Build history of the part. All positions in model axes, mm. Face numbers are marked on the shaded views. A direction names the side the tool comes from. Round coordinates to 2 decimals unless told otherwise and drop trailing zeros. Loops run counter-clockwise (first coordinate to the right, second up) from the corner with the lowest first, then second, coordinate; pieces in that order, holes last. Notation, with made-up numbers: M 7,5.5 L 55,5.5 A28 cw 55,24.5 Z; hole C 36.5,-39.5 d2. An arc over 180 degrees is marked long. Write each question's results on one line, items separated by ' | '. Start each with the question number.
Autodesk Inventor part; units mm, degrees
ref_plane "YZ Plane" through (0, 0, 0) normal (1, 0, 0) x (0, 1, 0)
ref_plane "XZ Plane" through (0, 0, 0) normal (0, 1, 0) x (-1, 0, 0)
ref_plane "XY Plane" through (0, 0, 0) normal (0, 0, 1) x (1, 0, 0)
sketch "Эскиз1" plane through (0, 0, 0) normal (0, 1, 0) x (-1, 0, 0)
  line L0 (0, 0) -> (0, -46)
  line L1 (0, 0) -> (10.9, 0)
  line L2 (10.9, 0) -> (10.9, -6.5)
  line L3 (10.9, -6.5) -> (9.2, -6.5)
  line L4 (9.2, -6.5) -> (9.2, -46)
  line L5 (9.2, -46) -> (0, -46)
  line L6 (0, 0) -> (-10.9, 0)
  line L7 (-10.9, 0) -> (-10.9, -6.5)
  line L8 (-10.9, -6.5) -> (-9.2, -6.5)
  line L9 (-9.2, -6.5) -> (-9.2, -46)
  line L10 (-9.2, -46) -> (0, -46)
  dimension "d1" = 6.5
  dimension "d2" = 46
  dimension "d3" = 18.4
  dimension "d4" = 21.8
extrude "Выдавливание1" add sketch "Эскиз1" along normal blind 1.5
chamfer "Фаска1" distance 2 angle 45 2 edges at (10.9, 0.75, 0) (-10.9, 0.75, 0)
chamfer "Фаска2" distance 1 angle 45 2 edges at (9.2, 0.75, -46) (-9.2, 0.75, -46)
sketch "Эскиз2" plane through (0, 1.5, 0) normal (0, 1, 0) x (1, 0, 0)
  line L0 (0, 0) -> (0, 46)
  line L1 (8.2, 46) -> (-8.2, 46)
  line L2 (-8.9, 0) -> (8.9, 0)
  point P0 (-8, 3.4)
  point P1 (8, 3.4)
  point P2 (-7, 44)
  point P3 (7, 44)
  dimension "d20" = 3.4
  dimension "d21" = 16
  dimension "d22" = 14
  dimension "d23" = 44
hole "Отверстие1" at (-8, 1.5, -3.4) at (8, 1.5, -3.4) at (-7, 1.5, -44) at (7, 1.5, -44) direction (0, -1, 0) diameter 2 end through all countersink diameter 3.2 countersink angle 90
sketch "Эскиз3" plane through (0, 0, 0) normal (0, -1, 0) x (1, 0, 0)
  line L0 (8.7, -6.9) -> (0, -6.9)
  line L1 (-8.9, 0) -> (8.9, 0)
  line L2 (8.7, -6.9) -> (8.7, -42)
  line L3 (10.9, -2) -> (10.9, -6.5)
  line L4 (8.7, -42) -> (6.2, -42)
  line L5 (4.2, -44) -> (4.2, -44)
  line L6 (4.2, -44) -> (0, -44)
  line L7 (8.7, -6.9) -> (5.8, -6.9)
  line L8 (0, 0) -> (0, -46)
  line L9 (8.2, -46) -> (-8.2, -46)
  arc A0 (6.2, -42) -> (4.2, -44) centre (6.2, -44) ccw
  line L10 (-8.7, -6.9) -> (0, -6.9)
  line L11 (-8.7, -6.9) -> (-8.7, -42)
  line L12 (-8.7, -42) -> (-6.2, -42)
  line L13 (-4.2, -44) -> (-4.2, -44)
  line L14 (-4.2, -44) -> (0, -44)
  line L15 (-8.7, -6.9) -> (-5.8, -6.9)
  arc A1 (-4.2, -44) -> (-6.2, -42) centre (-6.2, -44) ccw
  circle A2 centre (-7, -44) radius 1
  circle A3 centre (-8, -3.4) radius 1
  circle A4 centre (8, -3.4) radius 1
  circle A5 centre (7, -44) radius 1
  line L16 (-8.2, -46) -> (-9.2, -45)
  line L17 (8.2, -46) -> (-8.2, -46)
  line L18 (9.2, -45) -> (8.2, -46)
  line L19 (9.2, -6.5) -> (9.2, -45)
  line L20 (10.9, -6.5) -> (9.2, -6.5)
  line L21 (10.9, -2) -> (10.9, -6.5)
  line L22 (8.9, 0) -> (10.9, -2)
  line L23 (-8.9, 0) -> (8.9, 0)
  line L24 (-10.9, -2) -> (-8.9, 0)
  line L25 (-10.9, -6.5) -> (-10.9, -2)
  line L26 (-9.2, -6.5) -> (-10.9, -6.5)
  line L27 (-9.2, -45) -> (-9.2, -6.5)
  dimension "d24" = 6.9
  dimension "d25" = 2.2
  dimension "d26" = 42
  dimension "d27" = 44
  dimension "d28" = 6.7
  dimension "d30" = 2
extrude "Выдавливание2" add sketch "Эскиз3" along normal blind 0.8 contours L2 L4 A0 L6 L8 L0 | L8 L14 A1 L12 L11 L10
sketch "Эскиз5" plane through (0, -0.8, 0) normal (0, -1, 0) x (1, 0, 0)
  line L0 (-7.9, -42) -> (4.3, -42)
  line L1 (4.3, -42) -> (4.3, -8)
  line L2 (4.3, -8) -> (-7.9, -8)
  line L3 (-7.9, -8) -> (-7.9, -42)
  line L4 (-10.9, -6.5) -> (-10.9, -2)
  line L5 (9.2, -6.5) -> (9.2, -45)
  line L6 (-8.9, 0) -> (8.9, 0)
  line L7 (8.2, -46) -> (-8.2, -46)
  line L8 (-4.4, -42) -> (-4.4, -39)
  line L9 (-4.4, -39) -> (-7.9, -39)
  point P0 (0, 0)
  dimension "d33" = 3
  dimension "d35" = 8
  dimension "d36" = 4
  dimension "d40" = 31
  dimension "d41" = 3.5
  dimension "d55" = 12.2
extrude "Выдавливание3" cut sketch "Эскиз5" against normal blind 1.6 contours L8 L9 L3 L2 L1 L0
sketch "Эскиз6" plane through (0, 1.5, 0) normal (0, 1, 0) x (1, 0, 0)
  line L0 (-6.9, 9) -> (1.5, 9)
  line L1 (1.5, 9) -> (1.5, 35)
  line L2 (1.5, 35) -> (-6.9, 35)
  line L3 (-6.9, 35) -> (-6.9, 9)
  line L4 (-8.9, 0) -> (8.9, 0)
  line L5 (-9.2, 45) -> (-9.2, 6.5)
  line L6 (-10.9, 6.5) -> (-10.9, 2)
  line L7 (10.9, 2) -> (10.9, 6.5)
  point P0 (0, 0)
  dimension "d43" = 9
  dimension "d45" = 4
  dimension "d46" = 9.4
  dimension "d47" = 26
extrude "Выдавливание4" cut sketch "Эскиз6" against normal through all
fillet "Сопряжение2" radius 2 1 edges at (-0.05, 0.8, -42)
sketch "Эскиз7" plane through (0, 0, 0) normal (0, -1, 0) x (1, 0, 0)
  line L0 (-8.9, 0) -> (8.9, 0)
  line L1 (8.7, -6.9) -> (-8.7, -6.9)
  line L2 (6, 0) -> (-6, 0)
  line L3 (-6, 0) -> (-6, -6.9)
  line L4 (-6, -6.9) -> (6, -6.9)
  line L5 (6, -6.9) -> (6, 0)
  point P0 (0, 0)
  point P1 (0, 0)
  dimension "d51" = 12
extrude "Выдавливание5" add sketch "Эскиз7" along normal blind 2
properties part number "Case_top_new"
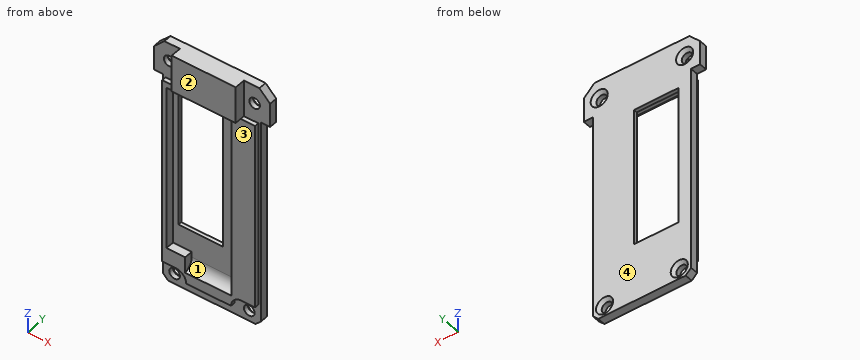
Item 1: Drill centre lines: line 1 along X through (y, z) = (0.4, -44); line 2 along X through (y, z) = (0.35, -3.4); line 3 along X through (y, z) = (1.25, -23). Where is each one in solid material? Low to high. Write a range as [from, to].
Item 2: Saw through at B-B, the plane z = -3.4. Give the cut face in (x, y), then the cut area to 3 significant figures.
Item 3: Mould opens along X. For the marked faces 1 and 2 say: released by +X, released by -X, zero draft, split by the parting line, or undercut.
Item 4: Saw through at C-C, the plane z = -8.5. Give the cut face in (x, y), then the cut area to 3 significant figures.
Item 5: Tool access for the marked faces 3 and 4: list every direction of +Z, -Z, +X, -X, +Y, -Y with a clear straight run to the whole face (end or side of a thin tool).
Item 6: Saw through at D-D, the plane y = -1.25. Give the cut face in (x, z).
Item 7: Saw through at A-A, the plane z = -14.5. Give the cut face in (x, y), then the cut area to 3 significant figures.
Item 8: Drop flat-ended pins along their axis: pin 1 (0.5 mm diameter, centred on y = 0, z = -25, fed in from -X); pin 2 (0.8 mm diameter, centred on y = 1, z = -25, fed in from +X); pin 3 (2.5 mm diameter, centred on x = 8, z = -3.4, fed in from +Y). Give the stop position or say it passes through.
Working result:
1) line 1: x = [-9.2, -8], [-6, 6], [8, 9.2] | line 2: x = [-10.9, -9], [-7, 7], [9, 10.9] | line 3: x = [-9.2, -6.9], [1.5, 9.2]
2) outline: M -10.9,0 L -9,0 L -9,0.9 L -9.6,1.5 L -10.9,1.5 Z; M -7,0 L -6,0 L -6,-2 L 6,-2 L 6,0 L 7,0 L 7,0.9 L 6.4,1.5 L -6.4,1.5 L -7,0.9 Z; M 9,0 L 10.9,0 L 10.9,1.5 L 9.6,1.5 L 9,0.9 Z | area: 50.0 mm²
3) face 1: undercut | face 2: zero draft
4) outline: M -9.2,0 L -8.7,0 L -8.7,-0.8 L -7.9,-0.8 L -7.9,0.8 L 4.3,0.8 L 4.3,-0.8 L 8.7,-0.8 L 8.7,0 L 9.2,0 L 9.2,1.5 L -9.2,1.5 Z | area: 22.0 mm²
5) face 3: -Z, +X, -X, -Y | face 4: +Z, -Z, +X, -X, +Y
6) outline: M -6,-6.9 L 6,-6.9 L 6,0 L -6,0 Z
7) outline: M -9.2,0 L -8.7,0 L -8.7,-0.8 L -7.9,-0.8 L -7.9,0.8 L -6.9,0.8 L -6.9,1.5 L -9.2,1.5 Z; M 1.5,0.8 L 4.3,0.8 L 4.3,-0.8 L 8.7,-0.8 L 8.7,0 L 9.2,0 L 9.2,1.5 L 1.5,1.5 Z | area: 16.1 mm²
8) pin 1: stops at x = -9.2 | pin 2: stops at x = 9.2 | pin 3: stops at y = 1.15
